The listing builds one solid part. Answer for the finished solid, in the listing's coordinates (mm). A direction names the side the tool comes from. Round coordinates to 2 decimals unless told otherwise and drop trailing zeros. Loops run counter-clockwise (first coordinate to the right, second up) from the corner with the lowest first, then second, coordinate; pieces in that order, holes last. Notation, with made-up numbers: (70, -3) - (126, -3) arc R8 ccw to (126, 9) - close; hole circle Ø7 at (54, -29). An arc over 180 degrees is marked (long way). One line per item, written item: value.
```python
from build123d import *

# Parameters (mm, degrees)
SKETCH_W        = 150
SKETCH_H        = 168
PAD_DEPTH       = 18
SKETCH001_W     = 150
SKETCH001_H     = 6
POCKET_DEPTH    = 6
SKETCH002_W     = 150
SKETCH002_H     = 6
POCKET001_DEPTH = 6


with BuildPart() as part:
    # Sketch → Pad (new body)
    with BuildSketch(Plane.XZ):
        with Locations((-75, 84)):
            Rectangle(SKETCH_W, SKETCH_H)
    extrude(amount=PAD_DEPTH)

    # Sketch001 (on Face6 of Pad) → Pocket (cut)
    with BuildSketch(Plane.XZ.offset(18)):
        with Locations((-75, 12)):
            Rectangle(SKETCH001_W, SKETCH001_H)
        with Locations((-75, 87)):
            Rectangle(SKETCH001_W, SKETCH001_H)
    extrude(amount=-POCKET_DEPTH, mode=Mode.SUBTRACT)

    # Sketch002 (on Face4 of Pocket) → Pocket001 (cut)
    with BuildSketch(Plane(origin=(0, 0, 0), x_dir=(1, 0, 0), z_dir=(0, 1, 0))):
        with Locations((-75, -12)):
            Rectangle(SKETCH002_W, SKETCH002_H)
        with Locations((-75, -87)):
            Rectangle(SKETCH002_W, SKETCH002_H)
    extrude(amount=-POCKET001_DEPTH, mode=Mode.SUBTRACT)


solid = part.part
```
1) Consider L1, parallel to Z at x = -23, y = -5.5. Determine where the line is inside the solid, lowest interval first.
Final values:
L1: 0 to 9, 15 to 84, 90 to 168
2) A cutting plane is placed at B-B on x = -71.5. Give the vertices of the cut face in (y, z), and give its area (3 significant figures).
Final values:
outline: (-18, 0) - (0, 0) - (0, 9) - (-6, 9) - (-6, 15) - (0, 15) - (0, 84) - (-6, 84) - (-6, 90) - (0, 90) - (0, 168) - (-18, 168) - (-18, 90) - (-12, 90) - (-12, 84) - (-18, 84) - (-18, 15) - (-12, 15) - (-12, 9) - (-18, 9) - close
area: 2,880 mm2
3) This flat-tipped pin is pushed along its axis until it touches: pin 1 Ø1.8 at (x, z) = (-41, 12) entering from +Y. Where does it stop, or does it pass through?
Final values:
pin 1: y = -6
4) For faces 1 (the flat face through (-76, -3, 9)), 2 (the flat face through (-76, 0, 5)), 3 (the flat face through (-76, -12, 87)), determine the directions among +Z, -Z, +X, -X, +Y, -Y from which every point of the face is accessible in a straight line to the end or side of a thin tool.
Final values:
face 1: +X, -X, +Y
face 2: +Z, -Z, +X, -X, +Y
face 3: +X, -X, -Y
5) For a pull along Z with two mould halves and no side action, classify faces 4 (the flat face through (-76, -3, 90)), 5 (the flat face through (-76, -9, 0)), 6 (the flat face through (-76, -9, 168)), 7 (the flat face through (-76, 0, 130)) as released by +Z, released by -Z, zero draft, split by the parting line, or undercut.
Final values:
face 4: undercut
face 5: released by -Z
face 6: released by +Z
face 7: zero draft
6) A cutting plane is placed at A-A on y = -14.5. Give the vertices of the cut face in (x, z).
Final values:
outline: (-150, 0) - (0, 0) - (0, 9) - (-150, 9) - close; (-150, 15) - (0, 15) - (0, 84) - (-150, 84) - close; (-150, 90) - (0, 90) - (0, 168) - (-150, 168) - close
7) A cutting plane is placed at C-C on z = 13. Give the vertices of the cut face in (x, y).
Final values:
outline: (-150, -12) - (0, -12) - (0, -6) - (-150, -6) - close
